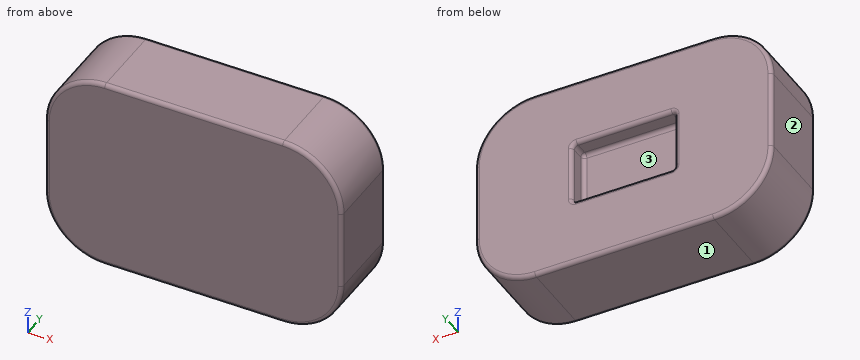
from build123d import *

# Parameters (mm, degrees)
SKETCH1_W           = 15
SKETCH1_H           = 10
BOSS_EXTRUDE1_DEPTH = 4
SKETCH2_W           = 5.2
SKETCH2_H           = 3.2
CUT_EXTRUDE1_DEPTH  = 1
FILLET1_R           = 3
FILLET2_R           = 0.2


with BuildPart() as part:
    # Sketch1 → Boss-Extrude1 (new body)
    with BuildSketch(Plane(origin=(0, 0, 0), x_dir=(1, 0, 0), z_dir=(0, 1, 0))):
        Rectangle(SKETCH1_W, SKETCH1_H)
    extrude(amount=BOSS_EXTRUDE1_DEPTH)

    # Sketch2 → Cut-Extrude1 (cut)
    with BuildSketch(Plane(origin=(0, 4, 0), x_dir=(1, 0, 0), z_dir=(0, 1, 0))):
        Rectangle(SKETCH2_W, SKETCH2_H)
    extrude(amount=-CUT_EXTRUDE1_DEPTH, mode=Mode.SUBTRACT)

    # Fillet1
    fillet1_edges = [part.edges().sort_by_distance(p)[0] for p in [
        (7.5, 2, 5),
        (-7.5, 2, 5),
        (-7.5, 2, -5),
        (7.5, 2, -5),
    ]]
    fillet(fillet1_edges, radius=FILLET1_R)

    # Fillet2
    fillet2_edges = [part.edges().sort_by_distance(p)[0] for p in [
        (2.6, 3, 0),
        (2.6, 3.5, -1.6),
        (0, 3, 1.6),
        (2.6, 3.5, 1.6),
        (-2.6, 3, 0),
        (-2.6, 3.5, 1.6),
        (0, 3, -1.6),
        (-2.6, 3.5, -1.6),
        (2.6, 4, 0),
        (0, 4, -1.6),
        (-2.6, 4, 0),
        (0, 4, 1.6),
        (-7.5, 0, 0),
        (-7.5, 4, 0),
        (7.5, 0, 0),
        (0, 0, 5),
        (0, 0, -5),
        (6.621320344, 0, 4.121320344),
        (-6.621320344, 0, 4.121320344),
        (6.621320344, 0, -4.121320344),
        (-6.621320344, 0, -4.121320344),
        (0, 4, -5),
        (7.5, 4, 0),
        (0, 4, 5),
        (6.621320344, 4, 4.121320344),
        (-6.621320344, 4, 4.121320344),
        (6.621320344, 4, -4.121320344),
        (-6.621320344, 4, -4.121320344),
    ]]
    fillet(fillet2_edges, radius=FILLET2_R)


solid = part.part
The model under review builds one solid part; all positions refer to its coordinate system, in mm. Face numbers are marked on the shaded views. Round coordinates to 2 decimals unless told otherwise and drop trailing zeros. Loops run counter-clockwise (first coordinate to the right, second up) from the corner with the lowest first, then second, coordinate; pieces in that order, holes last. Notation, with made-up numbers: (3, 45.25) -> (10, 45.25) arc R20 cw to (10, 84.25) -> close; hole circle Ø4 at (23, 49). An arc over 180 degrees is marked (long way). One line per question, with ' | ' between items. Start each with the question number.
Item 1: For pin 1 (0.8 mm diameter, centred on x = -1, z = 0, fed in from +Y), flat-tipped, find the tip position at first contact; note if it passes through.
Item 2: Add section A-A, the plane y = 0.4. Write out the cut boundary in (x, z), then the cut area to 3 significant figures.
Item 3: Wall thickness on line 1 along Z through (x, y) = (0.25, 3.2); line 2 along Y through (x, z) = (1, -1); line 3 along X through (y, z) = (3.55, -3.25): over which ranges is each line inside the solid? List them lowest first. Write a range as [from, to].
Item 4: Add section C-C, the plane z = 0.75. Write out the cut boundary in (x, y), then the cut area to 3 significant figures.
Item 5: Add section B-B, the plane x = 2.25. Write out the cut boundary in (y, z), then the cut area to 3 significant figures.
Item 6: Draft analysis for pull direction Z (two halves, no side actions). For the marked faces 1, 2 and 3, state which applies: +Z half, -Z half, draft (parallel to the pull), parting line (faces both ways), or undercut.
Return value:
1) pin 1: stops at y = 3
2) outline: (-7.5, -2) arc R3 ccw to (-4.5, -5) -> (4.5, -5) arc R3 ccw to (7.5, -2) -> (7.5, 2) arc R3 ccw to (4.5, 5) -> (-4.5, 5) arc R3 ccw to (-7.5, 2) -> close | area: 142 mm2
3) line 1: z = [-5, -1.6], [1.6, 5] | line 2: y = [0, 3] | line 3: x = [-7.23, 7.23]
4) outline: (-7.5, 0.2) arc R0.2 ccw to (-7.3, 0) -> (7.3, 0) arc R0.2 ccw to (7.5, 0.2) -> (7.5, 3.8) arc R0.2 ccw to (7.3, 4) -> (2.8, 4) arc R0.2 ccw to (2.6, 3.8) -> (2.6, 3.2) arc R0.2 cw to (2.4, 3) -> (-2.4, 3) arc R0.2 cw to (-2.6, 3.2) -> (-2.6, 3.8) arc R0.2 ccw to (-2.8, 4) -> (-7.3, 4) arc R0.2 ccw to (-7.5, 3.8) -> close | area: 54.8 mm2
5) outline: (0, -4.8) arc R0.2 ccw to (0.2, -5) -> (3.8, -5) arc R0.2 ccw to (4, -4.8) -> (4, -1.8) arc R0.2 ccw to (3.8, -1.6) -> (3.2, -1.6) arc R0.2 cw to (3, -1.4) -> (3, 1.4) arc R0.2 cw to (3.2, 1.6) -> (3.8, 1.6) arc R0.2 ccw to (4, 1.8) -> (4, 4.8) arc R0.2 ccw to (3.8, 5) -> (0.2, 5) arc R0.2 ccw to (0, 4.8) -> close | area: 36.8 mm2
6) face 1: -Z half | face 2: draft | face 3: undercut
